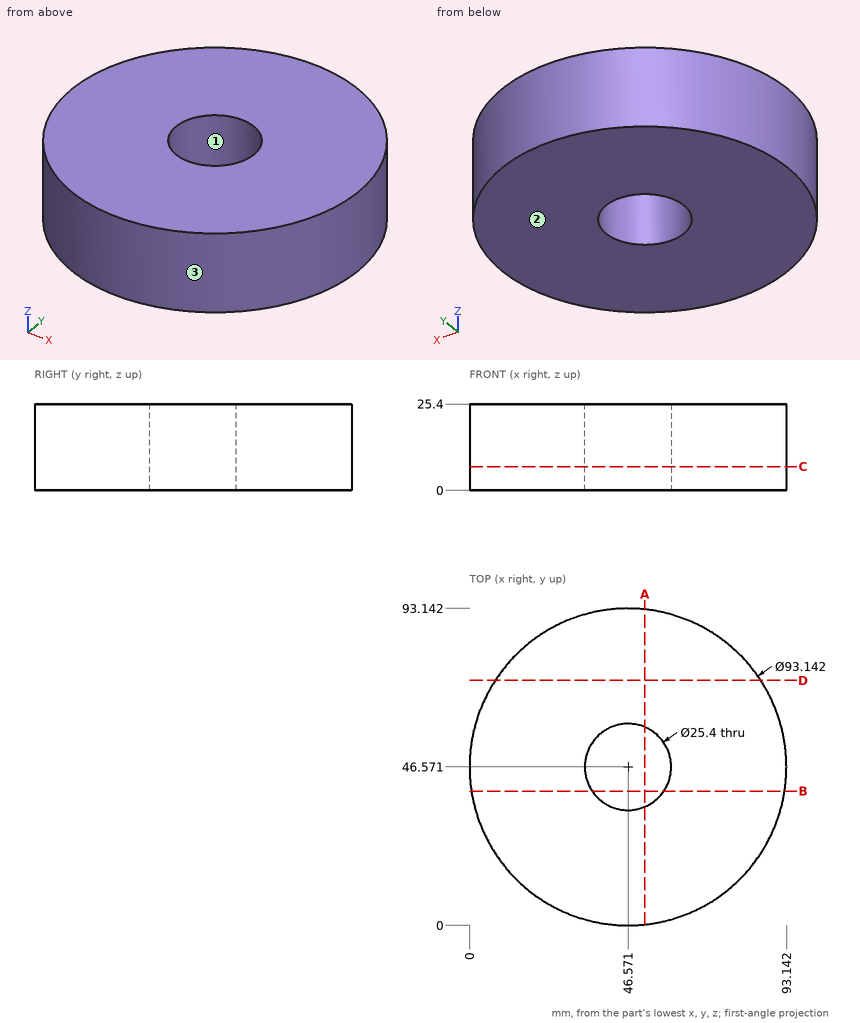
Geometry: see drawing. Coordinates: mm, zero at the bounding-box minimum. Round coordinates to 2 decimals unless told otherwise and drop trailing zeros. Loops run counter-clockwise (first coordinate to the right, second up) from the corner with the lowest first, then second, coordinate; pieces in that order, holes last. Notation, with made-up numbers: M 35.25,-29.75 L 67.25,-29.75 A23 cw 67.25,7.25 Z; hole C 50.25,67 d6. An arc over 180 degrees is marked long. Use a Markdown table: item, result. Add a question column.
1. Line query: line 1 (X direction, y = 55.5, z = 23.5) (1 decimal); line 2 (X direction, y = 56, z = 14.75) (1 decimal); line 3 (Y direction, x = 39, z = 6) (1 decimal). Output: solid intervals per line, ascending.
2. Section query A-A on x = 51.5. Return the cut outline in (y, z) (1 decimal).
3. Section query D-D on y = 72. Return the cut outline in (x, z) (1 decimal), then the cut area to 3 significant figures.
4. Contact query for flat-ended pins moving along their axis: P1, Ø8, axis at x = 38.5, z = 23, coming from the +Y side; P2, Ø2, axis at x = 53.5, z = 16, coming from the +Y side; P3, Ø10, axis at y = 17, z = 8, coming from the -X side. Output: stop coordinate, or through.
5. Section query B-B on y = 39.5. Return the cut outline in (x, z).
6. Section query C-C on z = 7. Return the cut outline in (x, y), then the cut area to 3 significant figures.
7. Mould query, pull axis Y, two halves, no side actions, for the marked faces 1, 2 and 3. Classes: pulls with the +Y half, pulls with the -Y half, needs draft (parallel to the pull), parting line crosses it, or undercut.
Reported:
| question | item | result |
|---|---|---|
| 1 | line 1 | x = 0.9 to 37.5, 55.6 to 92.3 |
| 1 | line 2 | x = 1 to 38.1, 55.1 to 92.2 |
| 1 | line 3 | y = 0.6 to 36.4, 56.8 to 92.5 |
| 2 | outline | M 0.3,0 L 34.9,0 L 34.9,25.4 L 0.3,25.4 Z; M 58.3,0 L 92.9,0 L 92.9,25.4 L 58.3,25.4 Z |
| 3 | outline | M 7.6,0 L 85.6,0 L 85.6,25.4 L 7.6,25.4 Z |
| 3 | area | 1,980 mm² |
| 4 | P1 | stops at y = 92.96 |
| 4 | P2 | stops at y = 92.76 |
| 4 | P3 | stops at x = 7.01 |
| 5 | outline | M 0.54,0 L 36.02,0 L 36.02,25.4 L 0.54,25.4 Z; M 57.12,0 L 92.6,0 L 92.6,25.4 L 57.12,25.4 Z |
| 6 | outline | C 46.57,46.57 d93.14; hole C 46.57,46.57 d25.4 |
| 6 | area | 6,310 mm² |
| 7 | face 1 | undercut |
| 7 | face 2 | needs draft |
| 7 | face 3 | parting line crosses it |
